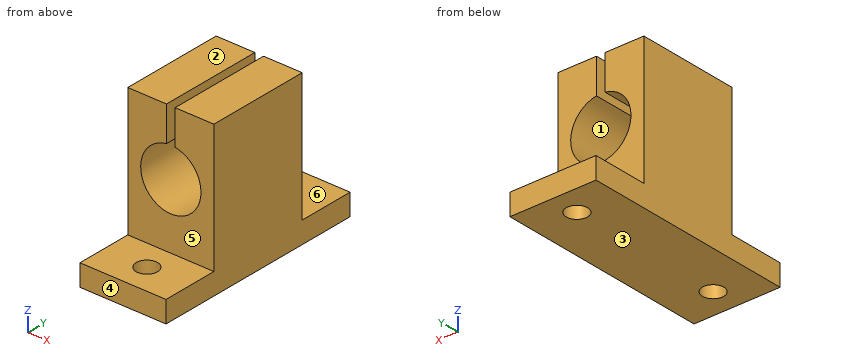
```python
from build123d import *

# Parameters (mm, degrees)
SKETCH020_W     = 20
SKETCH020_H     = 50
PAD011_DEPTH    = 5
SKETCH021_R     = 2.5
POCKET008_DEPTH = 5.001
SKETCH022_W     = 20
SKETCH022_H     = 24
PAD012_DEPTH    = 30
SKETCH023_R     = 7
POCKET009_DEPTH = 37.001
SKETCH024_W     = 2
SKETCH024_H     = 8.31
POCKET010_DEPTH = 37.001


with BuildPart() as part:
    # Sketch020 → Pad011 (new body)
    with BuildSketch(Plane.XY):
        Rectangle(SKETCH020_W, SKETCH020_H)
    extrude(amount=PAD011_DEPTH)

    # Sketch021 (on Face6 of Pad011) → Pocket008 (cut, through all)
    with BuildSketch(Plane.XY.offset(5)):
        with Locations((0, -18.5)):
            Circle(SKETCH021_R)
        with Locations((0, 18.5)):
            Circle(SKETCH021_R)
    extrude(amount=-POCKET008_DEPTH, mode=Mode.SUBTRACT)

    # Sketch022 (on Face5 of Pocket008) → Pad012 (join)
    with BuildSketch(Plane.XY.offset(5)):
        Rectangle(SKETCH022_W, SKETCH022_H)
    extrude(amount=PAD012_DEPTH)

    # Sketch023 (on Face12 of Pad012) → Pocket009 (cut, through all)
    with BuildSketch(Plane(origin=(0, 12, 0), x_dir=(-1, 0, 0), z_dir=(0, 1, 0))):
        with Locations((0, 20)):
            Circle(SKETCH023_R)
    extrude(amount=-POCKET009_DEPTH, mode=Mode.SUBTRACT)

    # Sketch024 (on Face12 of Pocket009) → Pocket010 (cut, through all)
    with BuildSketch(Plane(origin=(0, 12, 0), x_dir=(-1, 0, 0), z_dir=(0, 1, 0))):
        with Locations((0, 30.845)):
            Rectangle(SKETCH024_W, SKETCH024_H)
    extrude(amount=-POCKET010_DEPTH, mode=Mode.SUBTRACT)


solid = part.part
```
Model file for the job. Use its own axes, mm. Face numbers are marked on the shaded views. A direction names the side the tool comes from. Give positions to 0.01 mm unless a question says otherwise; leave off trailing zeros. Write each loop counter-clockwise with the first axis right and the second up, starting at its lowest first coordinate (ties: lowest second). Pieces come first, ordered by that corner, then holes. Notation, with made-up numbers: (55, 87) - (85, 87) arc R16 ccw to (85, 109) - close; hole circle Ø5 at (63.5, 33). An arc over 180 degrees is marked (long way). One line per question, with ' | ' between items. Start each with the question number.
(1) Slice it at C-C on y = -17. Write the cut outline in (x, z).
(2) Wall check: line 1 along Y through (x, z) = (0, 2.95); line 2 along X through (y, z) = (-2, 20); line 3 along X through (y, z) = (2, 33). Give the ranges that are in metal, low to high. Write a range as from..to.
(3) Slice it at A-A on z = 20. Write the cut outline in (x, y).
(4) 3-axis set-ups, long thin cutter, end or side, ignore diameter. For the marked faces 4, 5 and 6: which of +Z, -Z, +X, -X, +Y, -Y reach the whole face in a straight line?
(5) Slice it at D-D on x = 3.25. Write the cut outline in (y, z), plus the area to 3 significant figures.
(6) Pin check, flat tips, straight feed: P1, Ø8, axis at x = 0, y = -18.5, coming from the +Z side; P2, Ø3, axis at x = 6.5, z = 22.5, coming from the -Y side; P3, Ø11, axis at x = 0, z = 20, coming from the -Y side; P4, Ø2, axis at x = -5.5, z = 30.5, coming from the +Y side. Stop position of each tip, or through.
(7) Slice it at B-B on x = 0. Write the cut outline in (y, z), plus the area to 3 significant figures.
(8) Two-plate mould, pull along Z, no slides. Class the marked faces 1, 2 and 3: +Z half, -Z half, draft (parallel to the pull), parting line (faces both ways), or undercut.
Results below:
1) outline: (-10, 0) - (-2, 0) - (-2, 5) - (-10, 5) - close; (2, 0) - (10, 0) - (10, 5) - (2, 5) - close
2) line 1: -25..-21, -16..16, 21..25 | line 2: -10..-7, 7..10 | line 3: -10..-1, 1..10
3) outline: (-10, -12) - (-7, -12) - (-7, 12) - (-10, 12) - close; (7, -12) - (10, -12) - (10, 12) - (7, 12) - close
4) face 4: +Z, -Z, +X, -X, -Y | face 5: +Z, +X, -X, -Y | face 6: +Z, +X, -X, +Y
5) outline: (-25, 0) - (25, 0) - (25, 5) - (12, 5) - (12, 13.8) - (-12, 13.8) - (-12, 5) - (-25, 5) - close; (-12, 26.2) - (12, 26.2) - (12, 35) - (-12, 35) - close | area: 672 mm^2
6) P1: z = 5 | P2: y = -12 | P3: through | P4: y = 12
7) outline: (-25, 0) - (-21, 0) - (-21, 5) - (-25, 5) - close; (-16, 0) - (16, 0) - (16, 5) - (12, 5) - (12, 13) - (-12, 13) - (-12, 5) - (-16, 5) - close; (21, 0) - (25, 0) - (25, 5) - (21, 5) - close | area: 392 mm^2
8) face 1: undercut | face 2: +Z half | face 3: -Z half
